Autodesk Inventor part; units mm, degrees
ref_plane "YZ Plane" through (0, 0, 0) normal (1, 0, 0) x (0, 1, 0)
ref_plane "XZ Plane" through (0, 0, 0) normal (0, 1, 0) x (-1, 0, 0)
ref_plane "XY Plane" through (0, 0, 0) normal (0, 0, 1) x (1, 0, 0)
sketch "Skizze1" plane through (0, 0, 0) normal (0, 1, 0) x (-1, 0, 0)
  line L0 (35, 35) -> (-35, 35)
  line L1 (-35, 35) -> (-35, -35)
  line L2 (-35, -35) -> (35, -35)
  line L3 (35, -35) -> (35, 35)
  line L4 (0, 35) -> (0, -35) construction
  line L5 (35, 0) -> (-35, 0) construction
  point P0 (0, 0)
  point P1 (0, 0)
  dimension "d0" = 70
  dimension "d1" = 70
extrude "Extrusion1" add sketch "Skizze1" along normal blind 50
shell "Wandung1" thickness 4 removed faces 1 at (11.6667, 50, -11.6667)
sketch "Skizze2" plane through (35, 0, 35) normal (1, 0, 0) x (0, 0, -1)
  circle A0 centre (35, 27) radius 9.5
  line L0 (0, 0) -> (0, 50) construction
  line L1 (0, 0) -> (70, 0) construction
  line L2 (0, 50) -> (70, 0) construction
  line L3 (0, 50) -> (70, 50) construction
  line L4 (70, 50) -> (0, 0) construction
  point P0 (35, 0)
  point P1 (35, 25)
  point P2 (35, 25)
  dimension "d5" = 19
  dimension "d27" = 2
sketch "Skizze3" plane through (35, 0, -35) normal (0, 0, -1) x (-1, 0, 0)
  circle A0 centre (44, 25) radius 9.5
  line L0 (0, 0) -> (0, 50) construction
  line L1 (70, 0) -> (70, 50) construction
  line L2 (0, 50) -> (70, 0) construction
  line L3 (0, 50) -> (70, 50) construction
  line L4 (0, 0) -> (70, 50) construction
  point P0 (35, 0)
  point P1 (35, 25)
  point P2 (35, 25)
  dimension "d6" = 19
  dimension "d11" = 9
extrude "Extrusion2" cut sketch "Skizze3" against normal blind 95.5
extrude "Extrusion3" cut sketch "Skizze2" against normal blind 10
sketch "Skizze4" plane through (-31, 4, -31) normal (0, 1, 0) x (1, 0, 0)
  line L0 (62, -62) -> (0, -62)
  line L1 (62, 0) -> (0, 0)
  line L2 (62, -62) -> (46, -62)
  line L3 (46, -62) -> (46, 0)
  line L4 (46, 0) -> (62, 0)
  line L5 (62, 0) -> (62, -62)
  point P0 (31, -31)
  dimension "d12" = 16
extrude "Extrusion4" add sketch "Skizze4" along normal blind 11
sketch "Skizze5" plane through (-31, 15, -31) normal (0, 1, 0) x (1, 0, 0)
  line L0 (62, -62) -> (46, -62)
  line L1 (0, 0) -> (62, 0)
  line L2 (58, -62) -> (56, -62)
  line L3 (56, -62) -> (56, 0)
  line L4 (56, 0) -> (58, 0)
  line L5 (58, 0) -> (58, -62)
  line L6 (51, -62) -> (49, -62)
  line L7 (49, -62) -> (49, 0)
  line L8 (49, 0) -> (51, 0)
  line L9 (51, 0) -> (51, -62)
  line L10 (62, 0) -> (62, -62)
  line L11 (46, 0) -> (46, -62)
  line L12 (53.5, -62) -> (53.5, 0) construction
  point P0 (31, -31)
  point P1 (51, 0)
  point P2 (49, 0)
  point P3 (58, 0)
  dimension "d15" = 2
  dimension "d19" = 7.5
  dimension "d20" = 5
extrude "Extrusion5" cut sketch "Skizze5" against normal blind 3 contours L0 L3 L1 L5 | L0 L7 L1 L9
fillet "Rundung1" radius 1 4 edges at (27, 12, 0) (25, 12, 0) (20, 12, 0) (18, 12, 0)
sketch "Skizze6" plane through (-35, 0, -35) normal (-1, 0, 0) x (0, 0, 1)
  line L0 (70, 0) -> (70, 50) construction
  line L1 (70, 50) -> (0, 0) construction
  line L2 (0, 0) -> (70, 0) construction
  line L3 (70, 0) -> (0, 50) construction
  circle A0 centre (35, 25) radius 9.5
  point P0 (35, 0)
  dimension "d24" = 19
extrude "Extrusion6" cut sketch "Skizze6" against normal blind 10
properties part number "Hülle"
Can you work these out from the model? Positions are in its coordinate system, mm. A direction names the side the tool comes from. Round coordinates to 2 decimals unless told otherwise and drop trailing zeros. Order: outer loops, then holes, each group sorted by start corner. A loop starts at its lowest first (then second) coordinate and runs counter-clockwise, first axis right, second up. Notation, with made-up numbers: (37, 11) -> (83, 11) arc R22 cw to (83, 38) -> close; hole circle Ø4 at (72, -8). An arc over 180 degrees is marked (long way). Write each question's results on one line, items separated by ' | '. Start each with the question number.
Item 1: Thinking about a two-plate mould opening in X: for faces 1 (the flat face through (18, 14, 0)), 2 (the flat face through (-35, 19, -8)), 3 (the flat face through (0, 19, 35)), 4 (the flat face through (35, 19, -7)), which applies, +X half, -X half, draft (parallel to the pull), parting line (faces both ways), or undercut?
Item 2: If we section it at A-A, the plane z = 0: State how many separate pieces and enclosed holes the cut face has, then the cut area to 3 significant figures.
Item 3: Please list where these lines run through material, in increasing order: L1, parallel to Z at x = 0.5, y = 8; L2, parallel to Y at x = -8.5, z = -32.
Item 4: Which directions (+Z, -Z, +X, -X, +Y, -Y) give clear straight access to the entire face, cutting with the end or side of a thin tool? Please do faces 5 (the flat face through (27, 14, 0)), 6 (the flat face through (0, 0, 0)), 7 (the cylindrical face through (-33.028, 15.726, -2.059)), 8 (the cylindrical face through (33.028, 17.726, 2.059)).
Item 5: If we section it at B-B, the plane x = -9: Write out the boundary of the cut face in (y, z), then the cut area to 3 significant figures.
Item 6: If we section it at C-C, the plane y = 26: Write out the boundary of the cut face in (x, z).
Item 7: If we section it at D-D, the plane x = 11.5: Write out the boundary of the cut face in (y, z), then the cut area to 3 significant figures.
Item 8: Will these pins go through, and if not, where does the flat tip stop? pin 1 (22 mm diameter, centred on x = -9, y = 25, fed in from +Z); pin 2 (2 mm diameter, centred on x = 29, z = -6.5, fed in from +Y); pin 3 (10 mm diameter, centred on x = 9, z = -14.5, fed in from +Y).
Results:
1) face 1: undercut | face 2: -X half | face 3: draft | face 4: +X half
2) separate pieces: 3 | enclosed holes: 0 | area: 661 mm2
3) L1: z = -35 to -31, 31 to 35 | L2: y = 0 to 15.51, 34.49 to 50
4) face 5: +Y | face 6: +Z, -Z, +X, -X, -Y | face 7: -X | face 8: +X
5) outline: (0, -35) -> (15.5, -35) -> (15.5, -31) -> (4, -31) -> (4, 31) -> (15.5, 31) -> (15.5, 35) -> (0, 35) -> close; (34.5, -35) -> (50, -35) -> (50, -31) -> (34.5, -31) -> close; (34.5, 31) -> (50, 31) -> (50, 35) -> (34.5, 35) -> close | area: 496 mm2
6) outline: (-35, -35) -> (-18.45, -35) -> (-18.45, -31) -> (-31, -31) -> (-31, -9.45) -> (-35, -9.45) -> close; (-35, 9.45) -> (-31, 9.45) -> (-31, 31) -> (-18.45, 31) -> (-18.45, 35) -> (-35, 35) -> close; (0.45, -35) -> (35, -35) -> (35, -9.45) -> (31, -9.45) -> (31, -31) -> (0.45, -31) -> close; (0.45, 31) -> (31, 31) -> (31, 9.45) -> (35, 9.45) -> (35, 35) -> (0.45, 35) -> close
7) outline: (0, -35) -> (50, -35) -> (50, -31) -> (4, -31) -> (4, 31) -> (50, 31) -> (50, 35) -> (0, 35) -> close | area: 648 mm2
8) pin 1: stops at z = 35 | pin 2: stops at y = 15 | pin 3: stops at y = 4
